```python
from build123d import *

# Parameters (mm, degrees)
SKETCH1_W           = 4.7625
SKETCH1_H           = 4.7625
BOSS_EXTRUDE1_DEPTH = 20
SKETCH2_W           = 4
SKETCH2_H           = 4
CUT_EXTRUDE1_DEPTH  = 21.281536015
SKETCH3_R           = 0.79375
CUT_EXTRUDE2_DEPTH  = 10


with BuildPart() as part:
    # Sketch1 → Boss-Extrude1 (new body)
    with BuildSketch(Plane(origin=(0, 0, 0), x_dir=(0, 0, -1), z_dir=(1, 0, 0))):
        Rectangle(SKETCH1_W, SKETCH1_H)
    extrude(amount=BOSS_EXTRUDE1_DEPTH)

    # Sketch2 → Cut-Extrude1 (cut, through all)
    with BuildSketch(Plane.ZY):
        Rectangle(SKETCH2_W, SKETCH2_H)
    extrude(amount=-CUT_EXTRUDE1_DEPTH, mode=Mode.SUBTRACT)

    # Sketch3 → Cut-Extrude2 (cut)
    with BuildSketch(Plane(origin=(0, 2.38125, 0), x_dir=(1, 0, 0), z_dir=(0, 1, 0))):
        with Locations(Location((5, 0, 0), (0, 0, 270))):
            Circle(SKETCH3_R)
    extrude(amount=-CUT_EXTRUDE2_DEPTH, mode=Mode.SUBTRACT)


solid = part.part
```
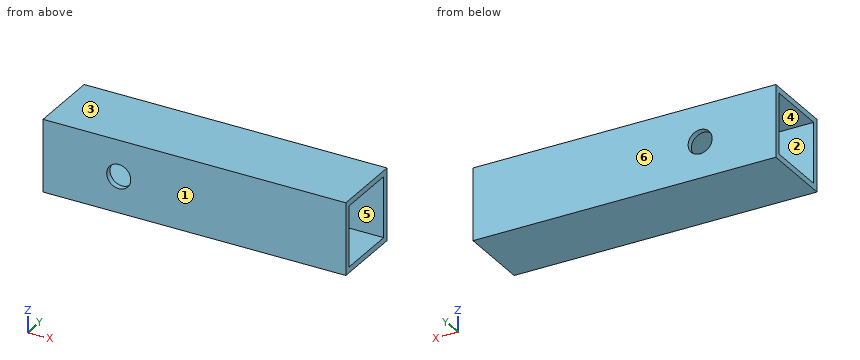
Geometry: final body of the model. Coordinates: model frame, mm. Face numbers are marked on the shaded views. A direction names the side the tool comes from. Round coordinates to 2 decimals unless told otherwise and drop trailing zeros. Order: outer loops, then holes, each group sorted by start corner. A loop starts at its lowest first (then second) coordinate and runs counter-clockwise, first axis right, second up. Notation, with made-up numbers: M 20.25,0.5 L 60.25,0.5 A25 ccw 60.25,19.5 Z; hole C -7,-18.75 d10. An arc over 180 degrees is marked long. Use one line per item in the form item = value. Start each with the question number.
Q1. Mould query, pull axis Y, two halves, no side actions, for the marked faces 1, 2, 3 and 4. Classes: +Y half, -Y half, draft (parallel to the pull), parting line (faces both ways), or undercut.
Q2. Cut plane B-B (z = 0). Return loops of the section in (x, y).
Q3. Cut plane C-C (z = -1.6). Return loops of the section in (x, y).
Q4. Cut plane A-A (x = 5). Return loops of the section in (y, z), and give its area (3 significant figures).
Q5. Pin query (flat end, axial travel): pin 1 Ø2.5 at (x, z) = (5, 0) entering from +Y. Return the tip coordinate at first contact, or that it passes through.
Q6. Access query for the marked faces 5 and 6. Directions: +Z, -Z, +X, -X, +Y, -Y. A direction counts if a zero-diameter tool reaches every point of the face in a straight line with its end or side. Return the directions, or none.
Q7. Material intervals for line 1 (Y direction, x = 14, z = 1.85); line 2 (X direction, y = 2.35, z = 0), sorted ascending. Write a range as [from, to].
Geometry results:
q1.face_1 = -Y half
q1.face_2 = undercut
q1.face_3 = draft
q1.face_4 = undercut
q2.outline = M 0,-2.38 L 4.21,-2.38 L 4.21,-2 L 0,-2 Z; M 0,2 L 4.21,2 L 4.21,2.38 L 0,2.38 Z; M 5.79,-2.38 L 20,-2.38 L 20,-2 L 5.79,-2 Z; M 5.79,2 L 20,2 L 20,2.38 L 5.79,2.38 Z
q3.outline = M 0,-2.38 L 20,-2.38 L 20,-2 L 0,-2 Z; M 0,2 L 20,2 L 20,2.38 L 0,2.38 Z
q4.outline = M -2.38,-2.38 L 2.38,-2.38 L 2.38,-0.79 L 2,-0.79 L 2,-2 L -2,-2 L -2,-0.79 L -2.38,-0.79 Z; M -2.38,0.79 L -2,0.79 L -2,2 L 2,2 L 2,0.79 L 2.38,0.79 L 2.38,2.38 L -2.38,2.38 Z
q4.area = 5.47 mm^2
q5.pin_1 = 2.38
q6.face_5 = +X, -X
q6.face_6 = +Z, -Z, +X, -X, +Y
q7.line_1 = [-2.38, -2], [2, 2.38]
q7.line_2 = [0, 4.21], [5.79, 20]
